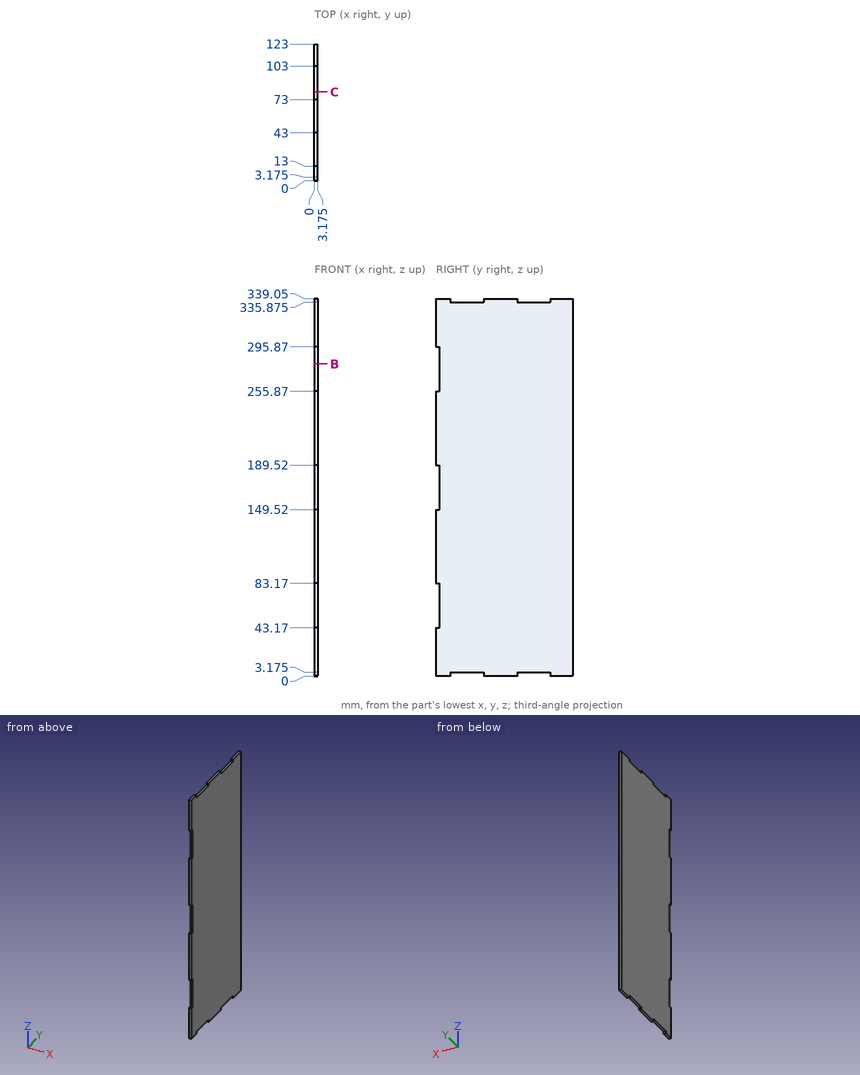
Source: three-view drawing plus pictorial views. Frame: mm from the lowest corner of the part. Round coordinates to 2 decimals unless told otherwise and drop trailing zeros. Loops run counter-clockwise (first coordinate to the right, second up) from the corner with the lowest first, then second, coordinate; pieces in that order, holes last. Notation, with made-up numbers: (-10, -36) - (38, -36) arc R9 ccw to (38, -25) - close; hole circle Ø7 at (-24, 33). An arc over 180 degrees is marked (long way). Write each question's results on one line, items separated by ' | '. Start each with the question number.
1) Line query: probe 1 along Z at (x, y) = (1.45, 32) (3 decimals); probe 2 along Y at (x, z) = (0.95, 271.5) (3 decimals). Output: solid intervals per line, ascending. Write a range as [from, to].
2) Cut plane C-C on y = 80. Return loops of the section in (x, z) (3 decimals), then the cut area to 3 significant figures.
3) Cut plane B-B on z = 280.5. Return loops of the section in (x, y) (3 decimals), then the cut area to 3 significant figures.
4) First-contact query: P1, Ø1, axis at x = 1, z = 58.5, coming from the -Y side (3 decimals). Flat tip, straight axial feed; report the tip coordinate or a pass-through.
Verdict:
1) probe 1: z = [3.175, 335.875] | probe 2: y = [3.175, 123]
2) outline: (0, 3.175) - (3.175, 3.175) - (3.175, 335.875) - (0, 335.875) - close | area: 1,060 mm2
3) outline: (0, 3.175) - (3.175, 3.175) - (3.175, 123) - (0, 123) - close | area: 380 mm2
4) P1: stops at y = 3.175
